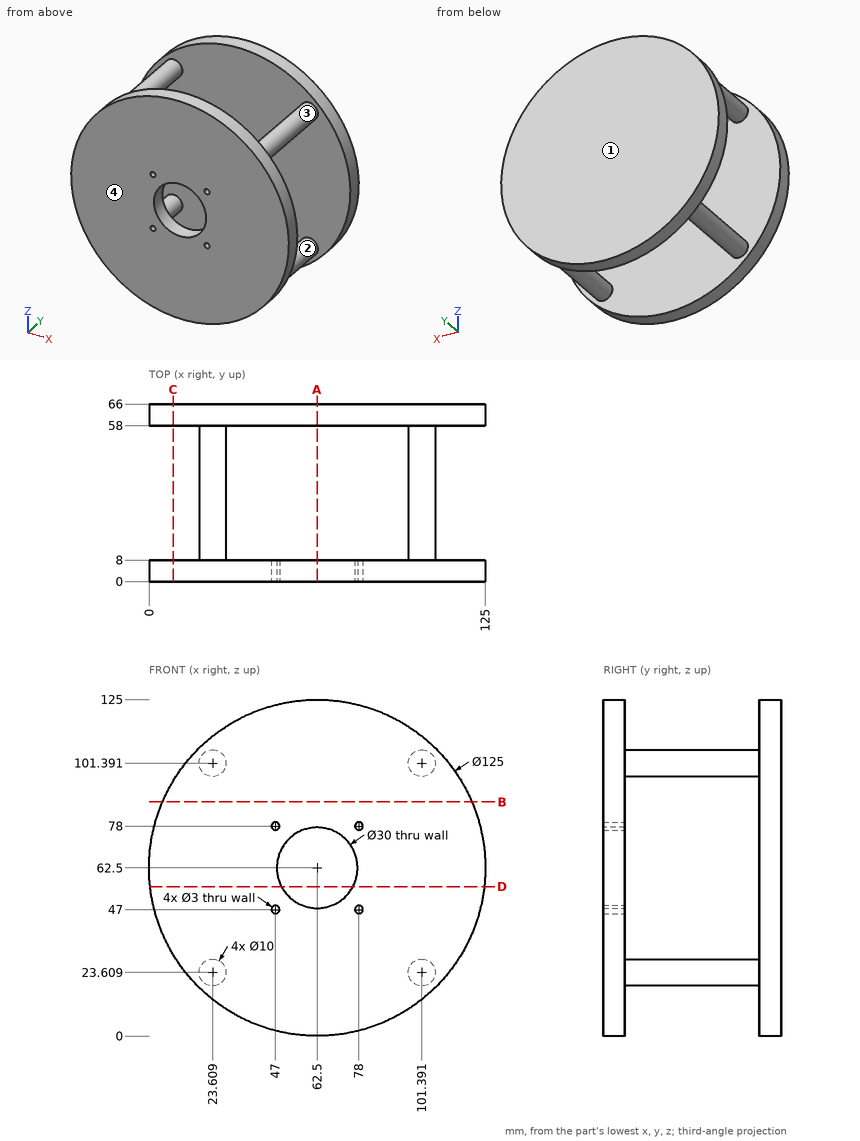
Geometry check sheet. Reference: drawing and pictorial views, mm from the part's lowest x, y, z. A direction names the side the tool comes from. Give positions to 0.01 mm unless a question says otherwise; leave off trailing zeros. Write each loop counter-clockwise with the first axis right and the second up, starting at its lowest first coordinate (ties: lowest second). Pieces come first, ordered by that corner, then holes. Notation, with made-up numbers: (-36, -29.75) - (-8, -29.75) arc R20 ccw to (-8, 2.25) - close; hole circle Ø10 at (-20.75, 87). An arc over 180 degrees is marked (long way). Use a Markdown table: item, result.
Q1. Draft check along Z on the marked faces 1 and 2. Enter one of: pulls with the +Z half, pulls with the -Z half, needs draft (parallel to the pull), parting line crosses it, or undercut.
Computed:
| item | result |
|---|---|
| face 1 | needs draft |
| face 2 | undercut |
Q2. Section check D-D, the plane z = 55.5. Enter the section's corners in (x, y), then the cut area to 3 significant figures.
Computed:
| item | result |
|---|---|
| outline | (0.39, 0) - (49.23, 0) - (49.23, 8) - (0.39, 8) - close; (0.39, 58) - (124.61, 58) - (124.61, 66) - (0.39, 66) - close; (75.77, 0) - (124.61, 0) - (124.61, 8) - (75.77, 8) - close |
| area | 1,780 mm² |
Q3. Go/stop test with flat-tipped pins: P1, Ø1.8, axis at x = 47, z = 78, coming from the -Y side; P2, Ø5, axis at y = 42, z = 96.5, coming from the +X side. Record where each tip stops, or that it passes through.
Computed:
| item | result |
|---|---|
| P1 | stops at y = 58 |
| P2 | stops at x = 105.78 |
Q4. Section check A-A, the plane x = 62.5. Enter the section's corners in (y, z).
Computed:
| item | result |
|---|---|
| outline | (0, 0) - (8, 0) - (8, 47.5) - (0, 47.5) - close; (0, 77.5) - (8, 77.5) - (8, 125) - (0, 125) - close; (58, 0) - (66, 0) - (66, 125) - (58, 125) - close |
Q5. Section check C-C, the plane x = 9. Enter the section's corners in (y, z).
Computed:
| item | result |
|---|---|
| outline | (0, 30.19) - (8, 30.19) - (8, 94.81) - (0, 94.81) - close; (58, 30.19) - (66, 30.19) - (66, 94.81) - (58, 94.81) - close |
Q6. Set-up check for the marked faces 3 and 4: record each of +Z, -Z, +X, -X, +Y, -Y from which the full face is reachable in a straight line by a thin tool's end or side.
Computed:
| item | result |
|---|---|
| face 3 | none |
| face 4 | +Z, -Z, +X, -X, -Y |
Q7. Thickness scan on L1, parallel to Y at x = 92, z = 85; L2, parallel to X at y = 3.75, z = 78. Record the ranges inside material, lowest first. Write a range as [from, to].
Computed:
| item | result |
|---|---|
| L1 | y = [0, 8], [58, 66] |
| L2 | x = [1.95, 45.5], [48.5, 76.5], [79.5, 123.05] |
Q8. Section check B-B, the plane z = 87. Enter the section's corners in (x, y).
Computed:
| item | result |
|---|---|
| outline | (5, 0) - (120, 0) - (120, 8) - (5, 8) - close; (5, 58) - (120, 58) - (120, 66) - (5, 66) - close |
